from build123d import *

# Parameters (mm, degrees)
F1_DEPTH = 3
F2_R     = 3
F4_D     = 1.6


with BuildPart() as f1:
    # F0 (on Front) → F1 (new body)
    with BuildSketch(Plane.XZ):
        with BuildLine():
            ThreePointArc((1, 0), (2, 1), (3, 0))
            Line((3, 0), (3, -1))
            Line((3, -1), (7, -1))
            Line((7, -1), (7, 2.5))
            Line((7, 2.5), (-7, 2.5))
            Line((-7, 2.5), (-7, -1))
            Line((-7, -1), (-3, -1))
            Line((-3, -1), (-3, 0))
            ThreePointArc((-3, 0), (-2, 1), (-1, 0))
            ThreePointArc((-1, 0), (0, 1), (1, 0))
        make_face()
    extrude(amount=F1_DEPTH)

    # F2
    f2_edges = [f1.edges().sort_by_distance(p)[0] for p in [
        (7, -1.5, 2.5),
        (-7, -1.5, 2.5),
    ]]
    fillet(f2_edges, radius=F2_R)

    # F4 (through all)
    with Locations(Plane(origin=(0, 0, -1), x_dir=(1, 0, 0), z_dir=(0, 0, -1))):
        with Locations((-5, 1.5), (5, 1.5)):
            Hole(F4_D / 2)


solid = f1.part
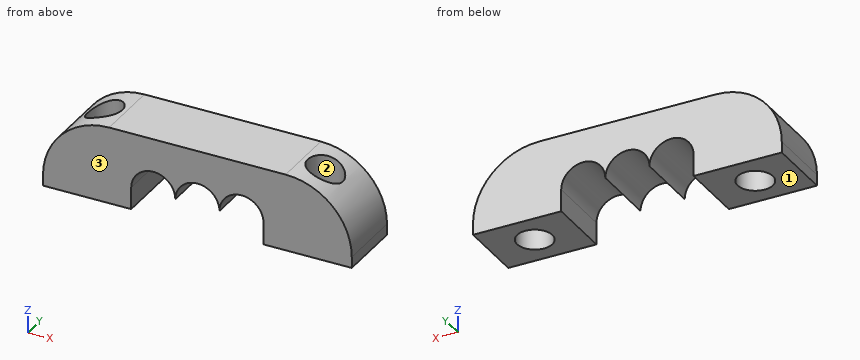
Geometry check sheet. Reference: the model listing, model coordinates, mm. Face numbers are marked on the shaded views. Round coordinates to 2 decimals unless told otherwise and drop trailing zeros. Write each loop counter-clockwise with the first axis right and the second up, starting at its lowest first coordinate (ties: lowest second). Pieces come first, ordered by that corner, then holes.
Item 1: Material ranges on line 1 along Y through (x, z) = (5, 1.7); line 2 along X through (y, z) = (-1.8, 1.25); line 3 along X through (y, z) = (-1.45, -0.6), recorded low to high.
Determined:
line 1: y = -3 to -2.3, -0.7 to 0
line 2: x = -6.44 to -5.74, -4.26 to 4.26, 5.74 to 6.44
line 3: x = -7 to -5.8, -4.2 to -3, 3 to 4.2, 5.8 to 7
Item 2: Section check C-C (x = -5). Record the boundary of the cut face in (y, z).
Determined:
outline: (-3, -1) - (-2.3, -1) - (-2.3, 2.33) - (-3, 2.33) - close; (-0.7, -1) - (0, -1) - (0, 2.33) - (-0.7, 2.33) - close
Item 3: Section check A-A (y = -1.5). Record the boundary of the cut face in (x, z).
Determined:
outline: (-7, -1) - (-5.8, -1) - (-5.8, 1.9) arc R3 ccw to (-7, -0.5) - close; (-4.2, -1) - (-3, -1) - (-3, 0) arc R1 cw to (-1, 0) arc R1 cw to (1, 0) arc R1 cw to (3, 0) - (3, -1) - (4.2, -1) - (4.2, 2.49) arc R3 ccw to (4, 2.5) - (-4, 2.5) arc R3 ccw to (-4.2, 2.49) - close; (5.8, -1) - (7, -1) - (7, -0.5) arc R3 ccw to (5.8, 1.9) - close
Item 4: Section check D-D (y = -0.9). Record the boundary of the cut face in (x, z), plus the area to 3 significant figures.
Determined:
outline: (-7, -1) - (-5.53, -1) - (-5.53, 2.08) arc R3 ccw to (-7, -0.5) - close; (-4.47, -1) - (-3, -1) - (-3, 0) arc R1 cw to (-1, 0) arc R1 cw to (1, 0) arc R1 cw to (3, 0) - (3, -1) - (4.47, -1) - (4.47, 2.46) arc R3 ccw to (4, 2.5) - (-4, 2.5) arc R3 ccw to (-4.47, 2.46) - close; (5.53, -1) - (7, -1) - (7, -0.5) arc R3 ccw to (5.53, 2.08) - close
area: 27.4 mm2
Item 5: Go/stop test with flat-tipped pins: pin 1 Ø1.5 at (y, z) = (-2, 0.5) entering from -X; pin 2 Ø1.4 at (x, y) = (5, -1.5) entering from -Z. Record where each tip stops, or that it passes through.
Determined:
pin 1: stops at x = -6.99
pin 2: passes through
Item 6: Section check B-B (z = 0.8). Record the boundary of the cut face in (x, y), plus the area to 3 significant figures.
Determined:
outline: (-6.7, -3) - (-2.6, -3) - (-2.6, 0) - (-6.7, 0) - close; (-1.4, -3) - (-0.6, -3) - (-0.6, 0) - (-1.4, 0) - close; (0.6, -3) - (1.4, -3) - (1.4, 0) - (0.6, 0) - close; (2.6, -3) - (6.7, -3) - (6.7, 0) - (2.6, 0) - close; hole circle Ø1.6 at (-5, -1.5); hole circle Ø1.6 at (5, -1.5)
area: 25.4 mm2
Item 7: Mould release check, pull along Y, two halves, no side actions. Record for the marked faces 1, 2 and 3: +Y half, -Y half, draft (parallel to the pull), parting line (faces both ways), or undercut.
Determined:
face 1: draft
face 2: undercut
face 3: -Y half
